Part model, mm, in its own coordinate system. Coordinates: 2 decimals unless noted, no trailing zeros. Write each loop counter-clockwise with the first axis right and the second up, starting at its lowest first coordinate (ties: lowest second). Pieces come first, ordered by that corner, then holes. Notation, with made-up numbers: (29.25, -8) -> (35.25, -8) arc R27 cw to (35.25, 24) -> close; hole circle Ø11 at (-21, 74.25). An arc over 180 degrees is marked (long way). Write item = value, one per line.
from build123d import *

# Parameters (mm, degrees)
F_8_32_TAPPED_HOLE1_D     = 3.4544
F_8_32_TAPPED_HOLE1_DEPTH = 11.43
F_8_32_TAPPED_HOLE1_TIP   = 1.037806461


with BuildPart() as part:
    # Sketch1 one side → Revolve1 (revolve)
    with BuildSketch(Plane.XY, mode=Mode.PRIVATE) as revolve1_sk:
        with BuildLine():
            Line((0, 3.175), (0, 0))
            Line((0, 0), (19.925615957, 0))
            ThreePointArc((19.925615957, 0), (19.771232823, 0.538397972), (19.355001042, 0.913174751))
            Line((19.355001042, 0.913174751), (4.953, 7.9375))
            Line((4.953, 7.9375), (4.953, 6.2865))
            ThreePointArc((4.953, 6.2865), (5.715, 5.5245), (4.953, 4.7625))
            Line((4.953, 4.7625), (3.175, 4.7625))
            Line((3.175, 4.7625), (3.175, 3.175))
            ThreePointArc((3.175, 3.175), (2.413, 2.413), (1.651, 3.175))
            Line((1.651, 3.175), (0, 3.175))
        make_face()
    revolve(revolve1_sk.sketch.rotate(Axis((-1.467236121, 0, 0), (1, 0, 0)), 90), axis=Axis((-1.467236121, 0, 0), (1, 0, 0)))

    # #8-32 Tapped Hole1
    with Locations(Plane.ZY):
        with Locations((0, 0)):
            Hole(F_8_32_TAPPED_HOLE1_D / 2, depth=F_8_32_TAPPED_HOLE1_DEPTH)
            with Locations((0, 0, -(F_8_32_TAPPED_HOLE1_DEPTH + F_8_32_TAPPED_HOLE1_TIP / 2))):  # 118° drill point
                Cone(0, F_8_32_TAPPED_HOLE1_D / 2, F_8_32_TAPPED_HOLE1_TIP, mode=Mode.SUBTRACT)


solid = part.part
Q1. Saw through at C-C on x = 15. Give the cut face in (y, z).
Model answer:
outline = circle Ø6.07 at (0, 0)
Q2. Saw through at D-D on x = 2.25. Give the cut face in (y, z).
Model answer:
outline = circle Ø4.86 at (0, 0); hole circle Ø3.45 at (0, 0)
Q3. Pin check, flat tips, straight feed: pin 1 (3 mm diameter, centred on y = -3, z = 4, fed in from -X) (3 decimals); pin 2 (1.5 mm diameter, centred on x = 3.5, y = -3.5, fed in from -Z); pin 3 (6 mm diameter, centred on x = 12, y = -3.5, fed in from +Z); pin 4 (1 mm diameter, centred on x = 15.5, y = 5, fed in from +Z). Stop position of each tip, or through.
Model answer:
pin_1 = 3.175
pin_2 = -3.89
pin_3 = 5.42
pin_4 = through
Q4. Saw through at A-A on x = 5.25. Give the cut face in (y, z).
Model answer:
outline = circle Ø15.59 at (0, 0); circle Ø9.65 at (0, 0); hole circle Ø12.45 at (0, 0); hole circle Ø3.45 at (0, 0)
Q5. Mould opens along Z. For faces 1 (the face through (13.65, 2.25, -2.93)), 2 (the face through (5.795, 1.713, 0.225)), 3 (the face through (0, 1.4, 1.4)) say: released by +Z, released by -Z, zero draft, split by the parting line, or undercut.
Model answer:
face_1 = split by the parting line
face_2 = undercut
face_3 = zero draft
Q6. Probe line 1 (Y direction, x = 3.5, z = 0); line 2 (Y direction, x = 5.5, z = 0) (3 decimals); line 3 (Y direction, x = 6.5, z = -1). List the from-to ranges inside material, lowest first. Write a range as from..to.
Model answer:
line_1 = -4.76..-1.73, 1.73..4.76
line_2 = -7.671..-6.055, -4.994..-1.727, 1.727..4.994, 6.055..7.671
line_3 = -7.11..-1.41, 1.41..7.11
Q7. Saw through at B-B on x = 8.75. Give the cut face in (y, z), and give its area (3 significant figures).
Model answer:
outline = circle Ø12.17 at (0, 0); hole circle Ø3.45 at (0, 0)
area = 107 mm²
